Autodesk Inventor part; units mm, degrees
ref_plane "YZ Plane" through (0, 0, 0) normal (1, 0, 0) x (0, 1, 0)
ref_plane "XZ Plane" through (0, 0, 0) normal (0, 1, 0) x (-1, 0, 0)
ref_plane "XY Plane" through (0, 0, 0) normal (0, 0, 1) x (1, 0, 0)
sketch "Sketch1" plane through (0, 0, 0) normal (0, 1, 0) x (-1, 0, 0)
  line L0 (98.75, 60) -> (-98.75, 60)
  line L1 (-98.75, 60) -> (-98.75, -60)
  line L2 (-98.75, -60) -> (98.75, -60)
  line L3 (98.75, -60) -> (98.75, 60)
  line L4 (98.75, 60) -> (-98.75, -60) construction
  line L5 (-98.75, 60) -> (98.75, -60) construction
  circle A0 centre (0, -40) radius 4
  circle A1 centre (0, 40) radius 4
  point P0 (0, 0)
  dimension "d0" = 197.5
  dimension "d1" = 120
  dimension "d2" = 8
  dimension "d3" = 20
  dimension "d4" = 8
  dimension "d5" = 80
extrude "Extrusion1" add sketch "Sketch1" along normal blind 5
sketch "Sketch2" plane through (0, 5, 0) normal (0, 1, 0) x (1, 0, 0)
  line L0 (-98.75, 60) -> (-98.75, -60)
  line L1 (98.75, -60) -> (98.75, 60)
  line L2 (98.75, 60) -> (-98.75, 60)
  line L3 (-98.75, -60) -> (98.75, -60)
  point P0 (0, 0)
  point P1 (-83.75, 20)
  point P2 (-83.75, -40)
  point P3 (83.75, -40)
  point P4 (83.75, 20)
  dimension "d8" = 15
  dimension "d9" = 15
  dimension "d17" = 15
  dimension "d18" = 15
  dimension "d19" = 40
  dimension "d20" = 40
  dimension "d21" = 20
  dimension "d22" = 20
hole "Hole1" at (83.75, 5, -20) at (-83.75, 5, -20) at (-83.75, 5, 40) at (83.75, 5, 40) direction (0, -1, 0) diameter 2 depth 4 tip angle 118 counterbore diameter 3.9 counterbore depth 2
properties part number "panel2"
For this review, take the finished solid that the model builds, in its own axes (mm). A direction names the side the tool comes from. Give positions to 0.01 mm unless a question says otherwise; leave off trailing zeros. Write each loop counter-clockwise with the first axis right and the second up, starting at its lowest first coordinate (ties: lowest second). Pieces come first, ordered by that corner, then holes. Notation, with made-up numbers: M -14,82.25 L 41,82.25 A32 ccw 41,113.25 Z; hole C 13.25,62 d11. An arc over 180 degrees is marked long. Answer as a JSON object with one key per item and string values. Group by question number.
Item 1: Draft analysis for pull direction X (two halves, no side actions). For faces 3 (the flat face through (98.75, 2, 1)), 4 (the cylindrical face through (82.106, 3.986, 41.048)), 5 (the flat face through (-1, 2, 60)), state which applies: +X half, -X half, draft (parallel to the pull), parting line (faces both ways), or undercut.
Item 2: Consider section A-A on z = -40. Write out the cut boundary in (x, y), plus the area to 4 significant figures.
Item 3: For probe 1 along Z at (x, y) = (-83.75, 1.45); probe 2 along Z at (x, y) = (83.75, 3.6); probe 3 along X at (y, z) = (3.95, -20), list the stretches that pass through material, from the lowest coordinate up. Write a range as [from, to].
Item 4: Consider section B-B on x = 0. Write out the cut boundary in (y, z), plus the area to 3 significant figures.
Item 5: Tool access review of faces 1 (the flat face through (1, 5, 1)), 2 (the cylindrical face through (-85.394, 3.986, 41.048)): name each direction out of +Z, -Z, +X, -X, +Y, -Y from which nothing blocks a thin tool from reaching the whole face with its end or side.
Item 6: For pin 1 Ø2 at (x, z) = (-84, 40.5) entering from +Y; pin 2 Ø5 at (x, z) = (0, 40) entering from +Y, all flat-tipped, find the tip position at first contact; note any pin that passes through.
Check result:
{
 "1": {"face 3": "+X half", "face 4": "undercut", "face 5": "draft"},
 "2": {"outline": "M -98.75,0 L -4,0 L -4,5 L -98.75,5 Z; M 4,0 L 98.75,0 L 98.75,5 L 4,5 Z", "area": "947.5 mm^2"},
 "3": {"probe 1": "z = [-60, -21], [-19, 39], [41, 60]", "probe 2": "z = [-60, -21.95], [-18.05, 38.05], [41.95, 60]", "probe 3": "x = [-98.75, -85.7], [-81.8, 81.8], [85.7, 98.75]"},
 "4": {"outline": "M 0,-60 L 5,-60 L 5,-44 L 0,-44 Z; M 0,-36 L 5,-36 L 5,36 L 0,36 Z; M 0,44 L 5,44 L 5,60 L 0,60 Z", "area": "520 mm^2"},
 "5": {"face 1": "+Z, -Z, +X, -X, +Y", "face 2": "+Y"},
 "6": {"pin 1": "stops at y = 3", "pin 2": "passes through"}
}
